Source: three-view drawing plus pictorial views. Frame: mm from the lowest corner of the part. A direction names the side the tool comes from. Round coordinates to 2 decimals unless told otherwise and drop trailing zeros. Loops run counter-clockwise (first coordinate to the right, second up) from the corner with the lowest first, then second, coordinate; pieces in that order, holes last. Notation, with made-up numbers: (-31, 43) -> (15, 43) arc R17 cw to (15, 72) -> close; hole circle Ø8 at (-15.75, 64). An arc over 180 degrees is marked (long way). One line per question, with ' | ' between items. Start each with the question number.
Q1. Mould query, pull axis Z, two halves, no side actions, for the marked faces 1 and 2. Classes: pulls with the +Z half, pulls with the -Z half, needs draft (parallel to the pull), parting line crosses it, or undercut.
Q2. Material intervals for L1, parallel to X at y = 11, z = 7.75; L2, parallel to Z at x = 15.5, y = 11.75; L3, parallel to X at y = 12, z = 15, sorted ascending.
Q3. Cut plane C-C on x = 40. Return loops of the section in (y, z), and give its area (3 significant figures).
Q4. Contact query for flat-ended pins moving along their axis: P1, Ø6, axis at y = 4, z = 4, coming from the +X side; P2, Ø4, axis at x = 20, y = 14.5, coming from the -Z side; P3, Ø10, axis at x = 29.5, y = 4, coming from the -Z side. Output: stop coordinate, or through.
Q5. Cut plane D-D on y = 17. Return loops of the section in (x, z), and give its area (3 significant figures).
Q6. Cut plane A-A on y = 12. Return loops of the section in (x, z), and give its area (3 significant figures).
Q7. Access query for the marked faces 3 and 4. Directions: +Z, -Z, +X, -X, +Y, -Y. A direction counts if a zero-diameter tool reaches every point of the face in a straight line with its end or side. Return the directions, or none.
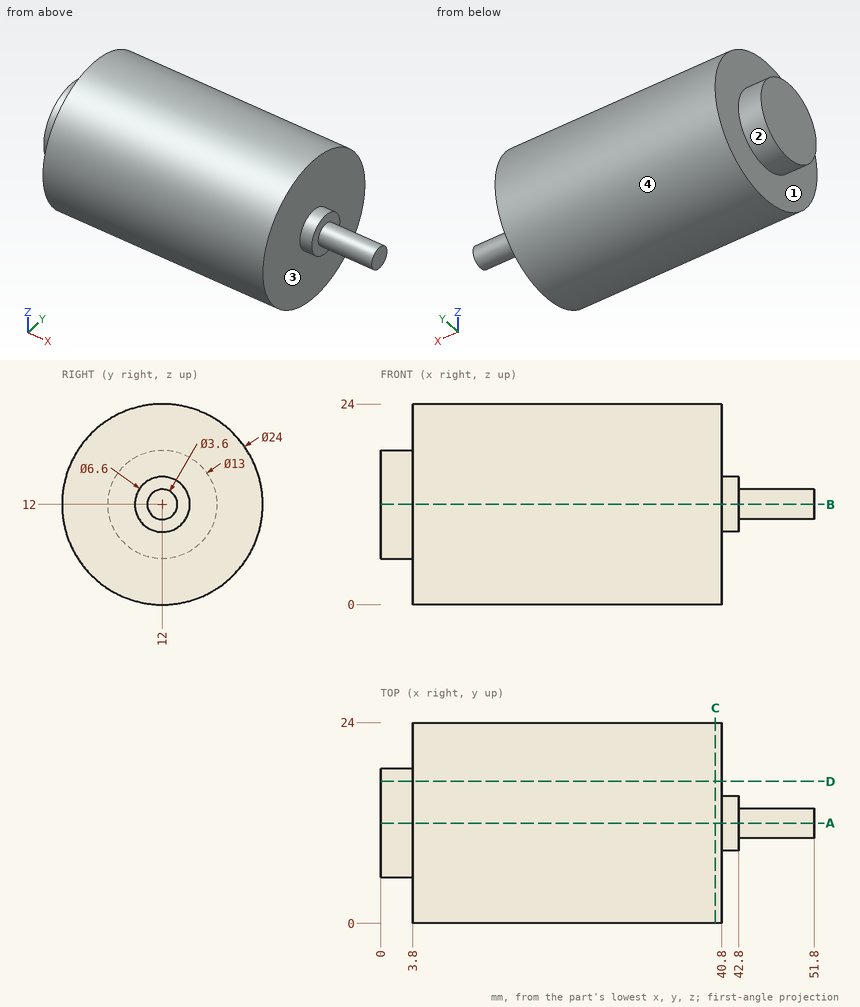
Results:
1) face 1: needs draft | face 2: parting line crosses it
2) L1: 0 to 40.8 | L2: 0 to 24 | L3: 0 to 42.8
3) outline: circle Ø24 at (12, 12) | area: 452 mm^2
4) P1: x = 40.8 | P2: z = 0.01 | P3: z = 0.38
5) outline: (0, 7.85) -> (3.8, 7.85) -> (3.8, 1.09) -> (40.8, 1.09) -> (40.8, 22.91) -> (3.8, 22.91) -> (3.8, 16.15) -> (0, 16.15) -> close | area: 839 mm^2
6) outline: (0, 5.5) -> (3.8, 5.5) -> (3.8, 0) -> (40.8, 0) -> (40.8, 8.7) -> (42.8, 8.7) -> (42.8, 10.2) -> (51.8, 10.2) -> (51.8, 13.8) -> (42.8, 13.8) -> (42.8, 15.3) -> (40.8, 15.3) -> (40.8, 24) -> (3.8, 24) -> (3.8, 18.5) -> (0, 18.5) -> close | area: 983 mm^2
7) face 3: +X | face 4: +X, -X
